Here's how the part is built. I have some questions about the finished solid (model axes, mm). Face numbers are marked on the shaded views. A direction names the side the tool comes from. Give positions to 0.01 mm unless a question says otherwise; leave off trailing zeros. Loops run counter-clockwise (first coordinate to the right, second up) from the corner with the lowest first, then second, coordinate; pieces in that order, holes last. Notation, with made-up numbers: (-17, 23.25) - (38, 23.25) arc R27 ccw to (38, 51.25) - close; hole circle Ø6 at (62, 8.25). An arc over 180 degrees is marked (long way). One line per item, written item: value. Start each with the question number.
```python
from build123d import *

# Parameters (mm, degrees)
ESQUISSE1_R        = 2
BOSS_EXTRU_1_DEPTH = 6


with BuildPart() as part:
    # Esquisse1 → Boss.-Extru.1 (new body)
    with BuildSketch(Plane.XY):
        with BuildLine():
            Line((-8.999739216, 15.2), (-5.999739216, 15.2))
            Line((-5.999739216, 15.2), (-5.999739216, 12.2))
            Line((-5.999739216, 12.2), (0.000260784, 12.2))
            Line((0.000260784, 12.2), (0, 2.2))
            Line((0, 2.2), (-5.999739216, 2.2))
            Line((-5.999739216, 2.2), (-5.999739216, -2.2))
            Line((-5.999739216, -2.2), (0.000260784, -2.2))
            Line((0.000260784, -2.2), (0.000260784, -12.2))
            Line((0.000260784, -12.2), (-5.999739216, -12.2))
            Line((-5.999739216, -12.2), (-5.999739216, -15.2))
            Line((-5.999739216, -15.2), (-8.999739216, -15.2))
            ThreePointArc((-8.999739216, -15.2), (-11.82816634, -14.028427125), (-12.999739216, -11.2))
            Line((-12.999739216, -11.2), (-12.999739216, -8.39638009))
            ThreePointArc((-12.999739216, -8.39638009), (-12.413952778, -6.982166528), (-10.999739216, -6.39638009))
            Line((-10.999739216, -6.39638009), (-10, -6.39638009))
            ThreePointArc((-10, -6.39638009), (-8.585786438, -5.810593653), (-8, -4.39638009))
            Line((-8, -4.39638009), (-8, 4.39638009))
            ThreePointArc((-8, 4.39638009), (-8.585786438, 5.810593653), (-10, 6.39638009))
            Line((-10, 6.39638009), (-10.999739216, 6.39638009))
            ThreePointArc((-10.999739216, 6.39638009), (-12.413952778, 6.982166528), (-12.999739216, 8.39638009))
            Line((-12.999739216, 8.39638009), (-12.999739216, 11.2))
            ThreePointArc((-12.999739216, 11.2), (-11.82816634, 14.028427125), (-8.999739216, 15.2))
        make_face()
        with Locations((-8.999739216, 11.2)):
            Circle(ESQUISSE1_R, mode=Mode.SUBTRACT)
        with Locations((-8.999739216, -11.2)):
            Circle(ESQUISSE1_R, mode=Mode.SUBTRACT)
    extrude(amount=BOSS_EXTRU_1_DEPTH)


solid = part.part
```
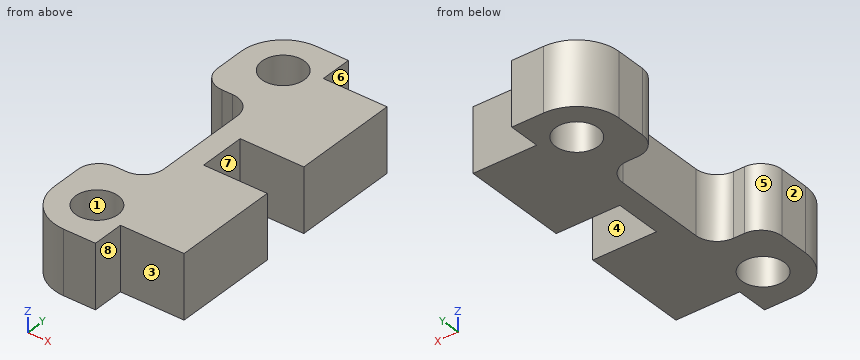
(1) Will these pins go through, and if not, where does the flat tip stop? pin 1 (0.9 mm diameter, centred on y = -14.5, z = 3, fed in from +X); pin 2 (0.8 mm diameter, centred on x = -10.5, z = 2.5, fed in from +Y); pin 3 (1 mm diameter, centred on x = -2, z = 1, fed in from +Y).
(2) If we section it at B-B on y = 12.5: List the corners of the cut face in (x, z) for me.
(3) If we section it at A-A on x = -1: List the corners of the cut face in (y, z) for me.
(4) For the marked faces 5, 6, 7 and 8, which set-ups out of +Z, -Z, +X, -X, +Y, -Y let a thin tool reach every point of the face, with its end or its side?
(5) If we section it at C-C on z = 5.6: List the corners of the cut face in (x, y) for me.
(6) Please list where these lines run through material, in increasing order: probe 1 along Y at (x, z) = (-5.25, 2.7); probe 2 along X at (y, z) = (-4, 3.8); probe 3 along X at (y, z) = (10.5, 2.85). Write a range as from..to.
(7) If we section it at D-D on x = -8.5: List the corners of the cut face in (y, z) for me, plus the area to 3 significant figures.
(8) If we mould it in two halves opening along Y, with no side actions, what happens to the marked faces 1, 2, 3 and 4? For each: pulls with the +Y half, pulls with the -Y half, needs draft (parallel to the pull), parting line crosses it, or undercut.
Found:
1. pin 1: x = -6
1. pin 2: y = 15.05
1. pin 3: y = 12.2
2. outline: (-12.78, 0) - (-10.52, 0) - (-10.52, 6) - (-12.78, 6) - close; (-7.48, 0) - (-6, 0) - (-6, 6) - (-7.48, 6) - close
3. outline: (-12.2, 0) - (-2.2, 0) - (-2.2, 6) - (-12.2, 6) - close; (2.2, 0) - (12.2, 0) - (12.2, 6) - (2.2, 6) - close
4. face 5: +Z, -Z, -X
4. face 6: +Z, -Z, +X, +Y
4. face 7: +Z, -Z, +X
4. face 8: +Z, -Z, +X, -Y
5. outline: (-13, -11.2) arc R4 ccw to (-9, -15.2) - (-6, -15.2) - (-6, -12.2) - (0, -12.2) - (0, -2.2) - (-6, -2.2) - (-6, 2.2) - (0, 2.2) - (0, 12.2) - (-6, 12.2) - (-6, 15.2) - (-9, 15.2) arc R4 ccw to (-13, 11.2) - (-13, 8.4) arc R2 ccw to (-11, 6.4) - (-10, 6.4) arc R2 cw to (-8, 4.4) - (-8, -4.4) arc R2 cw to (-10, -6.4) - (-11, -6.4) arc R2 ccw to (-13, -8.4) - close; hole circle Ø4 at (-9, -11.2); hole circle Ø4 at (-9, 11.2)
6. probe 1: -12.2..-2.2, 2.2..12.2
6. probe 2: -8..0
6. probe 3: -13..-10.87, -7.13..0
7. outline: (-15.2, 0) - (-13.14, 0) - (-13.14, 6) - (-15.2, 6) - close; (-9.26, 0) - (-5.72, 0) - (-5.72, 6) - (-9.26, 6) - close; (5.72, 0) - (9.26, 0) - (9.26, 6) - (5.72, 6) - close; (13.14, 0) - (15.2, 0) - (15.2, 6) - (13.14, 6) - close
7. area: 67.3 mm^2
8. face 1: undercut
8. face 2: needs draft
8. face 3: pulls with the -Y half
8. face 4: undercut
